```python
from build123d import *

# Parameters (mm, degrees)
EXTRUDE1_DEPTH          = 15.875
EXTRUDE1_DEPTH_BACK     = 15.875
SKETCH1_R               = 2.413
SKETCH8_OUTSIDE_W       = 134.808
SKETCH8_OUTSIDE_H       = 136.282
SKETCH8_OUTSIDE_R       = 4.7625
EXTRUDE4_DEPTH          = 33.572776689
EXTRUDE4_DRAFT          = -60
MIRROR1_COPY_1_SKETCH_W = 134.808
MIRROR1_COPY_1_SKETCH_H = 136.282
MIRROR1_COPY_1_SKETCH_R = 4.7625
MIRROR1_COPY_1_DEPTH    = 33.572776689
MIRROR1_COPY_1_DRAFT    = -60


with BuildPart() as part:
    # Sketch1 → Extrude1 (new, two sides: drawn at the far end of the back side and taken through both)
    with BuildSketch(Plane.XY.offset(-EXTRUDE1_DEPTH_BACK)):
        Polygon((0, 5.499261314), (-4.7625, 2.749630657), (-4.7625, -2.749630657), (0, -5.499261314), (4.7625, -2.749630657), (4.7625, 2.749630657), align=None)
        Circle(SKETCH1_R, mode=Mode.SUBTRACT)
    extrude(amount=EXTRUDE1_DEPTH + EXTRUDE1_DEPTH_BACK)

    # Extrude3 cone 1 section (through the dimple's axis) → Extrude3 (revolve, cut)
    with BuildSketch(Plane(origin=(0, 0, -15.875), x_dir=(0, 1, 0), z_dir=(1, 0, 0))):
        Polygon((0, 0), (2.4638, 0), (0, 2.642102028), align=None)
    extrude3 = revolve(axis=Axis((0, 0, -15.875), (0, 0, 1)), mode=Mode.SUBTRACT)


with BuildPart() as extrude4_tool:
    # Sketch8 outside → Extrude4 (with draft: the straight prism first)
    with BuildSketch(Plane(origin=(0, 0, -15.875), x_dir=(-1, 0, 0), z_dir=(0, 0, -1))):
        Rectangle(SKETCH8_OUTSIDE_W, SKETCH8_OUTSIDE_H)
        Circle(SKETCH8_OUTSIDE_R, mode=Mode.SUBTRACT)
    extrude(amount=-EXTRUDE4_DEPTH)
    # Extrude4: the draft: its side faces are tilted about the plane it starts from
    extrude4_sides = [extrude4_tool.faces().sort_by_distance(p)[0] for p in [
        (0, -68.141, 0.911388345),
        (-67.404, 0, 0.911388345),
        (0, 68.141, 0.911388345),
        (67.404, 0, 0.911388345),
        (4.7625, 0, 0.911388345),
    ]]
    draft(extrude4_sides, Plane(origin=(0, 0, -15.875), x_dir=(-1, 0, 0), z_dir=(0, 0, -1)), EXTRUDE4_DRAFT)


with BuildPart() as part_1:
    add(part.part)

    # Extrude4: cut by extrude4_tool
    add(extrude4_tool.part, mode=Mode.SUBTRACT)

    # Mirror1: Extrude3 across plane
    add(extrude3.mirror(Plane.XY), mode=Mode.SUBTRACT)


with BuildPart() as mirror1_copy_1_tool:
    # Mirror1 copy 1 sketch → Mirror1 copy 1 (with draft: the straight prism first)
    with BuildSketch(Plane(origin=(0, 0, 15.875), x_dir=(-1, 0, 0), z_dir=(0, 0, 1))):
        Rectangle(MIRROR1_COPY_1_SKETCH_W, MIRROR1_COPY_1_SKETCH_H)
        Circle(MIRROR1_COPY_1_SKETCH_R, mode=Mode.SUBTRACT)
    extrude(amount=-MIRROR1_COPY_1_DEPTH)
    # Mirror1 copy 1: the draft: its side faces are tilted about the plane it starts from
    mirror1_copy_1_sides = [mirror1_copy_1_tool.faces().sort_by_distance(p)[0] for p in [
        (0, -68.141, -0.911388345),
        (-67.404, 0, -0.911388345),
        (0, 68.141, -0.911388345),
        (67.404, 0, -0.911388345),
        (4.7625, 0, -0.911388345),
    ]]
    draft(mirror1_copy_1_sides, Plane(origin=(0, 0, 15.875), x_dir=(-1, 0, 0), z_dir=(0, 0, 1)), MIRROR1_COPY_1_DRAFT)


with BuildPart() as part_2:
    add(part_1.part)

    # Mirror1 copy 1: cut by mirror1_copy_1_tool
    add(mirror1_copy_1_tool.part, mode=Mode.SUBTRACT)


solid = part_2.part
```
The listing builds one solid part. Answer for the finished solid, in the listing's coordinates (mm). Coordinates: 2 decimals unless noted, no trailing zeros. Loops run counter-clockwise (first coordinate to the right, second up) from the corner with the lowest first, then second, coordinate; pieces in that order, holes last. Notation, with made-up numbers: M 20,12 L 50,12 A20 ccw 50,49 Z; hole C 77,64 d10. An arc over 180 degrees is marked long. Answer as a JSON object with one key per item and string values. Group by question number.
Item 1: Consider L1, parallel to X at y = 0, z = -2; L2, parallel to Y at x = 2, z = 2.5; L3, parallel to Y at x = 0.25, z = 2. Determine where each line is inside the solid, lowest interval first.
Item 2: Section A-A (z = 8.5) is taken. Write down the section's boundary in (x, y), and give its area (3 significant figures).
Item 3: Each of these flat-tipped pins is pushed along its axis until it touches: P1, Ø2, axis at x = 3.5, z = -4, coming from the -Y side; P2, Ø1.5, axis at x = -1, z = 2.5, coming from the -Y side; P3, Ø3, axis at x = 3.5, z = 3, coming from the +Y side. Where does it stop, or does it pass through?
Solved:
{
 "1": {"L1": "x = -4.76 to -2.41, 2.41 to 4.76", "L2": "y = -4.34 to -1.35, 1.35 to 4.34", "L3": "y = -5.35 to -2.4, 2.4 to 5.35"},
 "2": {"outline": "M -4.76,-2.75 L 0,-5.5 L 4.76,-2.75 L 4.76,2.75 L 0,5.5 L -4.76,2.75 Z; hole C 0,0 d4.83", "area": "60.3 mm2"},
 "3": {"P1": "stops at y = -4.06", "P2": "stops at y = -5.35", "P3": "stops at y = 4.34"}
}
